```python
from build123d import *

# Parameters (mm, degrees)
BOX015_W     = 25.5
BOX015_H     = 2
BOX015_DEPTH = 10
BOX016_W     = 2
BOX016_H     = 8
BOX016_DEPTH = 10
BOX017_W     = 2
BOX017_H     = 64
BOX017_DEPTH = 10
BOX014_W     = 25.5
BOX014_H     = 2
BOX014_DEPTH = 10
BOX013_W     = 2
BOX013_H     = 91
BOX013_DEPTH = 10
BOX011_W     = 18.5
BOX011_H     = 88
BOX011_DEPTH = 5
BOX010_W     = 21.5
BOX010_H     = 91
BOX010_DEPTH = 5


with BuildPart() as frame_top:
    # Box015 → Box015 (new body)
    with BuildSketch(Plane(origin=(-2, 91, 0), x_dir=(1, 0, 0), z_dir=(0, 0, 1))):
        with Locations((12.75, 1)):
            Rectangle(BOX015_W, BOX015_H)
    extrude(amount=BOX015_DEPTH)


with BuildPart() as frame_right_bottom:
    # Box016 → Box016 (new body)
    with BuildSketch(Plane(origin=(21.5, 0, 0), x_dir=(1, 0, 0), z_dir=(0, 0, 1))):
        with Locations((1, 4)):
            Rectangle(BOX016_W, BOX016_H)
    extrude(amount=BOX016_DEPTH)


with BuildPart() as frame_right_top:
    # Box017 → Box017 (new body)
    with BuildSketch(Plane(origin=(21.5, 27, 0), x_dir=(1, 0, 0), z_dir=(0, 0, 1))):
        with Locations((1, 32)):
            Rectangle(BOX017_W, BOX017_H)
    extrude(amount=BOX017_DEPTH)


with BuildPart() as frame_bottom:
    # Box014 → Box014 (new body)
    with BuildSketch(Plane(origin=(-2, -2, 0), x_dir=(1, 0, 0), z_dir=(0, 0, 1))):
        with Locations((12.75, 1)):
            Rectangle(BOX014_W, BOX014_H)
    extrude(amount=BOX014_DEPTH)


with BuildPart() as frame:
    # Box013 → Box013 (new body)
    with BuildSketch(Plane(origin=(-2, 0, 0), x_dir=(1, 0, 0), z_dir=(0, 0, 1))):
        with Locations((1, 45.5)):
            Rectangle(BOX013_W, BOX013_H)
    extrude(amount=BOX013_DEPTH)

    # Fusion: union frame_bottom
    add(frame_bottom.part)

    # Fusion001: union frame_right_top
    add(frame_right_top.part)

    # Fusion002: union frame_right_bottom
    add(frame_right_bottom.part)

    # Fusion003: union frame_top
    add(frame_top.part)


with BuildPart() as cube005:
    # Box011 → Box011 (new body)
    with BuildSketch(Plane(origin=(1.5, 1.5, 0), x_dir=(1, 0, 0), z_dir=(0, 0, 1))):
        with Locations((9.25, 44)):
            Rectangle(BOX011_W, BOX011_H)
    extrude(amount=BOX011_DEPTH)


with BuildPart() as fusion004:
    # Box010 → Box010 (new body)
    with BuildSketch(Plane.XY):
        with Locations((10.75, 45.5)):
            Rectangle(BOX010_W, BOX010_H)
    extrude(amount=BOX010_DEPTH)

    # Cut006: cut Cube005
    add(cube005.part, mode=Mode.SUBTRACT)

    # Fusion004: union frame
    add(frame.part)


solid = fusion004.part
```
Can you work these out from the model? Positions are in its coordinate system, mm. A direction names the side the tool comes from. Give positions to 0.01 mm unless a question says otherwise; leave off trailing zeros. Order: outer loops, then holes, each group sorted by start corner. A loop starts at its lowest first (then second) coordinate and runs counter-clockwise, first axis right, second up. Notation, with made-up numbers: (53.25, 26) - (77.25, 26) arc R26 cw to (77.25, 49) - close; hole circle Ø10 at (62, -29). An arc over 180 degrees is marked (long way). Use a Markdown table: item, result. Add a question column.
Q1. If we section it at A-A on x = 17.5: Write out the boundary of the cut face in (y, z), plus the area to 3 significant figures.
Q2. If we mould it in two halves opening along X, with no side actions, what happens to faces 6 (the flat face through (23.5, 3, 5)), 7 (the flat face through (11, 93, 5)), 8 (the flat face through (0, 45, 7))? For each: released by +X, released by -X, zero draft, split by the parting line, or undercut.
Q3. I'm going to push flat-ended pins straight in: pin 1 (1.5 mm diameter, centred on y = 18, z = 2, fed in from +X); pin 2 (6 mm diameter, centred on x = 4, y = 9, fed in from +Z). Where does each tip first touch, or does it pass through?
Q4. If we section it at B-B on y = 82.5: Write out the boundary of the cut face in (x, z).
Q5. Please list where these lines run through material, in increasing order: line 1 along X through (y, z) = (78.5, 5.5); line 2 along Y through (x, z) = (7.25, 7.25); line 3 along Y through (x, z) = (3.5, 1.5).
Q6. If we section it at C-C on z = 3.25: Write out the boundary of the cut face in (x, y), plus the area to 4 significant figures.
Q7. On a 3-axis mill with a long thin cutter (end or side, diameter ignored), from which of +Z, -Z, +X, -X, +Y, -Y can I reach the whole of each face in a straight line? I mean faces 1 (the flat face through (-2, 45, 5)), 2 (the flat face through (20, 45, 2)), 3 (the flat face through (22, 8, 5)), 4 (the flat face through (11, 0, 7)), 5 (the flat face through (11, -2, 5)). Say none if no direction works.
Answers follow:
| question | item | result |
|---|---|---|
| 1 | outline | (-2, 0) - (1.5, 0) - (1.5, 5) - (0, 5) - (0, 10) - (-2, 10) - close; (89.5, 0) - (93, 0) - (93, 10) - (91, 10) - (91, 5) - (89.5, 5) - close |
| 1 | area | 55.0 mm^2 |
| 2 | face 6 | released by +X |
| 2 | face 7 | zero draft |
| 2 | face 8 | undercut |
| 3 | pin 1 | stops at x = 21.5 |
| 3 | pin 2 | stops at z = 5 |
| 4 | outline | (-2, 0) - (1.5, 0) - (1.5, 5) - (0, 5) - (0, 10) - (-2, 10) - close; (20, 0) - (23.5, 0) - (23.5, 10) - (21.5, 10) - (21.5, 5) - (20, 5) - close |
| 5 | line 1 | x = -2 to 0, 21.5 to 23.5 |
| 5 | line 2 | y = -2 to 0, 91 to 93 |
| 5 | line 3 | y = -2 to 1.5, 89.5 to 93 |
| 6 | outline | (-2, -2) - (23.5, -2) - (23.5, 8) - (21.5, 8) - (21.5, 27) - (23.5, 27) - (23.5, 93) - (-2, 93) - close; hole (1.5, 1.5) - (20, 1.5) - (20, 89.5) - (1.5, 89.5) - close |
| 6 | area | 756.5 mm^2 |
| 7 | face 1 | +Z, -Z, -X, +Y, -Y |
| 7 | face 2 | +Z, -Z |
| 7 | face 3 | +Z, -Z, +X |
| 7 | face 4 | +Z |
| 7 | face 5 | +Z, -Z, +X, -X, -Y |
